Geometry check sheet. Reference: the model listing, model coordinates, mm. Round coordinates to 2 decimals unless told otherwise and drop trailing zeros. Write each loop counter-clockwise with the first axis right and the second up, starting at its lowest first coordinate (ties: lowest second). Pieces come first, ordered by that corner, then holes. Notation, with made-up numbers: M 59,69.25 L 109,69.25 A23 ccw 109,79.25 Z; hole C 70,-15 d6. An arc over 180 degrees is marked long. One line per item, written item: value. Start each with the question number.
1. Depth check by flat-ended pin: P1, Ø0.8, axis at x = -20.5, z = 1, coming from the +Y side (3 decimals). Enter the tip coordinate at first touch or a pass-through.
2. Section check A-A (y = 0). Record the boundary of the cut face in (x, z) (1 decimal).
3. Scan lines: probe 1 along X at (y, z) = (2, 0.25); probe 2 along X at (y, z) = (1, 0.1); probe 3 along X at (y, z) = (-1.5, 1.35). Record each from-to range of solid material in increasing order. Write a range as [from, to].
4. Section check C-C (y = 19.05). Record the boundary of the cut face in (x, z), and give its area (3 significant figures).
5. Section check D-D (x = -19.5). Record the boundary of the cut face in (y, z) (1 decimal).
6. Section check B-B (z = 1.15). Count the separate pieces of the cut face and the enclosed holes in it, and give its area (3 significant figures).
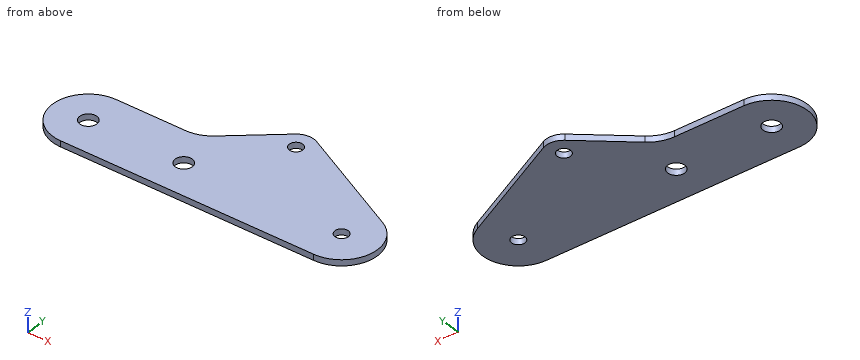
from build123d import *

# Parameters (mm, degrees)
SKETCH1_R           = 2.286
SKETCH1_R_2         = 1.778
BOSS_EXTRUDE1_DEPTH = 1.5875


with BuildPart() as part:
    # Sketch1 → Boss-Extrude1 (new body)
    with BuildSketch(Plane.XY):
        with BuildLine():
            Line((-3.929505469, -9.525), (38.1, -9.525))
            ThreePointArc((38.1, -9.525), (47.363212424, -2.217773791), (42.413639839, 8.492239772))
            Line((42.413639839, 8.492239772), (13.269319919, 23.296119886))
            ThreePointArc((13.269319919, 23.296119886), (10.554316452, 23.779676244), (8.026471806, 22.677373187))
            Line((8.026471806, 22.677373187), (-4.764567756, 11.795253626))
            ThreePointArc((-4.764567756, 11.795253626), (-7.648450959, 10.11056254), (-10.936624143, 9.525))
            Line((-10.936624143, 9.525), (-29.329505469, 9.525))
            ThreePointArc((-29.329505469, 9.525), (-38.854505469, 0), (-29.329505469, -9.525))
            Line((-29.329505469, -9.525), (-3.929505469, -9.525))
        make_face()
        with Locations((-3.929505469, 0)):
            Circle(SKETCH1_R, mode=Mode.SUBTRACT)
        with Locations((38.1, 0)):
            Circle(SKETCH1_R_2, mode=Mode.SUBTRACT)
        with Locations((11.1125, 19.05)):
            Circle(SKETCH1_R_2, mode=Mode.SUBTRACT)
        with Locations((-29.329505469, 0)):
            Circle(SKETCH1_R, mode=Mode.SUBTRACT)
    extrude(amount=BOSS_EXTRUDE1_DEPTH)


solid = part.part
Result sheet:
1. P1: stops at y = 9.525
2. outline: M -38.9,0 L -31.6,0 L -31.6,1.6 L -38.9,1.6 Z; M -27,0 L -6.2,0 L -6.2,1.6 L -27,1.6 Z; M -1.6,0 L 36.3,0 L 36.3,1.6 L -1.6,1.6 Z; M 39.9,0 L 47.6,0 L 47.6,1.6 L 39.9,1.6 Z
3. probe 1: x = [-38.64, -30.44], [-28.22, -5.04], [-2.82, 47.41]
3. probe 2: x = [-38.8, -31.39], [-27.27, -5.99], [-1.87, 36.63], [39.57, 47.57]
3. probe 3: x = [-38.74, -31.05], [-27.6, -5.65], [-2.2, 37.15], [39.05, 47.51]
4. outline: M 3.76,0 L 9.33,0 L 9.33,1.59 L 3.76,1.59 Z; M 12.89,0 L 21.63,0 L 21.63,1.59 L 12.89,1.59 Z
4. area: 22.7 mm2
5. outline: M -9.5,0 L 9.5,0 L 9.5,1.6 L -9.5,1.6 Z
6. separate pieces: 1
6. enclosed holes: 4
6. area: 1,880 mm2
